Build history of the part. All positions in model axes, mm. Face numbers are marked on the shaded views. A direction names the side the tool comes from. Coordinates: 2 decimals unless noted, no trailing zeros. Order: outer loops, then holes, each group sorted by start corner. A loop starts at its lowest first (then second) coordinate and runs counter-clockwise, first axis right, second up. Notation, with made-up numbers: M 55,-18 L 113,-18 A18 cw 113,6 Z; hole C -7.75,49.25 d3. An arc over 180 degrees is marked long. Use a Markdown table: item, result. Add a question column.
Autodesk Inventor part; units mm, degrees
ref_plane "YZ Plane" through (0, 0, 0) normal (1, 0, 0) x (0, 1, 0)
ref_plane "XZ Plane" through (0, 0, 0) normal (0, 1, 0) x (-1, 0, 0)
ref_plane "XY Plane" through (0, 0, 0) normal (0, 0, 1) x (1, 0, 0)
sketch "Sketch5" plane through (0, 0, 0) normal (0, 0, 1) x (1, 0, 0)
  line L0 (0, 0) -> (-60, 0)
  line L1 (-60, 0) -> (-60, 60)
  line L2 (-60, 60) -> (0, 60)
  line L3 (0, 60) -> (0, 0)
  dimension "d55" = 60
  dimension "d56" = 60
extrude "Extrusion4" add sketch "Sketch5" along normal blind 35.4
sketch "Sketch6" plane through (0, 0, 0) normal (1, 0, 0) x (0, 0, -1)
  line L0 (-35.4, 60) -> (-35.4, 0)
  line L1 (-35.4, 60) -> (-25.4, 60)
  line L2 (-25.4, 60) -> (-25.4, 50)
  line L3 (-25.4, 50) -> (-35.4, 50)
  line L4 (-35.4, 50) -> (-35.4, 60)
  line L5 (-25.4, 50) -> (-9.4, 50)
  line L6 (-9.4, 50) -> (-9.4, 29.6)
  line L7 (-9.4, 29.6) -> (-25.4, 29.6)
  line L8 (-25.4, 29.6) -> (-25.4, 50)
  point P0 (0, 0)
  dimension "d61" = 10
  dimension "d62" = 10
  dimension "d65" = 16
  dimension "d66" = 20.4
extrude "Extrusion5" cut sketch "Sketch6" against normal blind 50 contours L5 L6 L7 L8
fillet "Fillet5" radius 2 6 edges at (-30, 60, 35.4) (-25, 29.6, 25.4) (-25, 50, 25.4) (-60, 30, 35.4) (-60, 0, 17.7) (-60, 60, 17.7)
properties part number "Clasp"
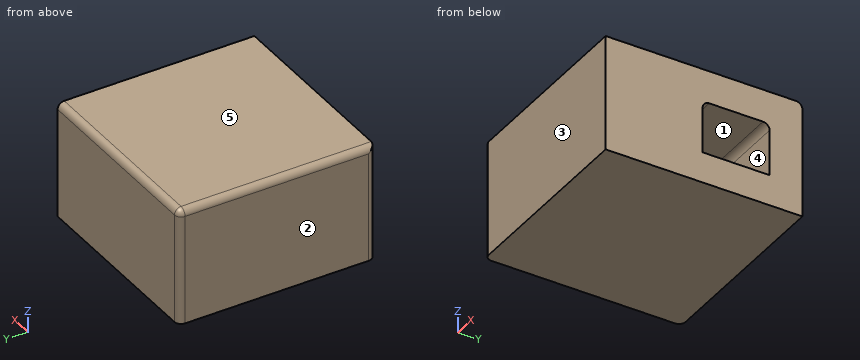
(1) Drill centre lines: line 1 along Z through (x, y) = (-21.5, 42.5); line 2 along Y through (x, z) = (-48, 21); line 3 along X through (y, z) = (47, 24.5). Where is each one in solid material? Low to high. Write a range as from..to.
(2) Which spindle directions (+Z, -Z, +X, -X, +Y, -Y) get a long thin tool onto all of the face, cutting with end or side? Do the marked faces 1 and 2. Say none if no direction does.
(3) Slice it at A-A on x = -25. Give the cut face in (y, z), and give its area (3 significant figures).
(4) Drop flat-ended pins along their axis: P1, Ø4, axis at x = -30.5, z = 16.5, coming from the -Y side; P2, Ø5, axis at y = 37, z = 14, coming from the +X side. Give the stop position or say it passes through.
(5) Slice it at B-B on y = 32.5. Give the cut face in (x, z), and give its area (3 significant figures).
(6) Mould opens along Z. For the marked faces 3, 4 and 5 say: released by +Z, released by -Z, zero draft, split by the parting line, or undercut.
(7) Slice it at C-C on z = 12.5. Give the cut face in (x, y).
Solutions:
| question | item | result |
|---|---|---|
| 1 | line 1 | 0..9.4, 25.4..35.4 |
| 1 | line 2 | 0..29.6, 50..60 |
| 1 | line 3 | -60..-50 |
| 2 | face 1 | +X |
| 2 | face 2 | +Z, -Z, -X, +Y, -Y |
| 3 | outline | M 0,0 L 60,0 L 60,33.4 A2 ccw 58,35.4 L 0,35.4 Z; hole M 29.6,9.4 L 50,9.4 L 50,23.4 A2 ccw 48,25.4 L 31.6,25.4 A2 ccw 29.6,23.4 Z |
| 3 | area | 1,800 mm² |
| 4 | P1 | y = 0 |
| 4 | P2 | x = -50 |
| 5 | outline | M -60,0 L 0,0 L 0,9.4 L -50,9.4 L -50,25.4 L 0,25.4 L 0,35.4 L -58,35.4 A2 ccw -60,33.4 Z |
| 5 | area | 1,320 mm² |
| 6 | face 3 | zero draft |
| 6 | face 4 | undercut |
| 6 | face 5 | released by +Z |
| 7 | outline | M -60,2 A2 ccw -58,0 L 0,0 L 0,29.6 L -50,29.6 L -50,50 L 0,50 L 0,60 L -58,60 A2 ccw -60,58 Z |
